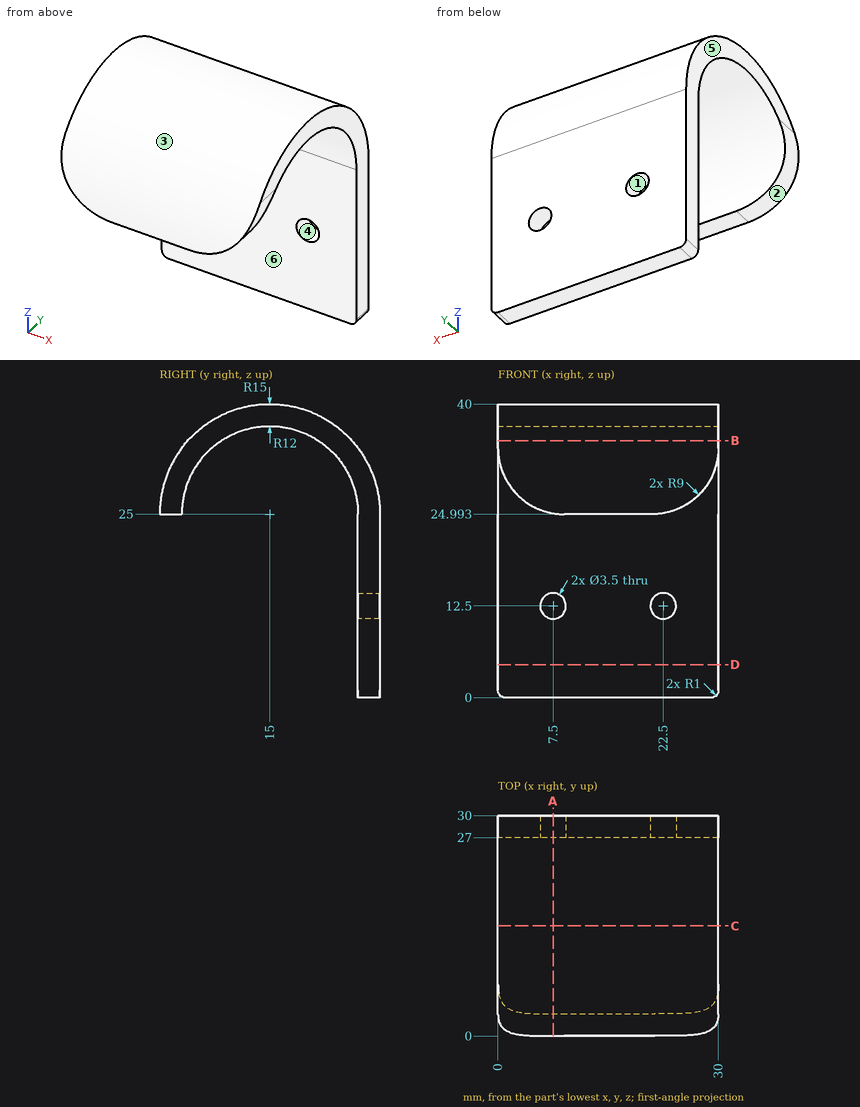
Source: three-view drawing plus pictorial views. Frame: mm from the lowest corner of the part. A direction names the side the tool comes from. Round coordinates to 2 decimals unless told otherwise and drop trailing zeros. Loops run counter-clockwise (first coordinate to the right, second up) from the corner with the lowest first, then second, coordinate; pieces in that order, holes last.
Q1. Pull-direction query (X, two-part tool) for the marked faces 1, 2, 3 and 4; classes: released by +X, released by -X, zero draft, split by the parting line, or undercut.
Q2. Section B-B on z = 35. Return loops of the section in (x, y).
Q3. Pin query (flat end, axial travel): P1, Ø12, axis at x = 24, z = 11.5, coming from the -Y side; P2, Ø1.5, axis at x = 15.5, y = 2, coming from the -Z side; P3, Ø1, axis at y = 25.5, z = 22, coming from the -X side; P4, Ø8, axis at x = 11.5, z = 35.5, coming from the -Y side. Return the tip coordinate at first contact, or that it passes through.
Q4. Section C-C on y = 15. Return loops of the section in (x, z).
Q5. Section A-A on x = 7.5. Return loops of the section in (y, z), plus the area to 3 significant figures.
Q6. Section D-D on z = 4.5. Return loops of the section in (x, y), plus the area to 3 significant figures.
Q7. Access query for the marked faces 5 and 6. Directions: +Z, -Z, +X, -X, +Y, -Y. A direction counts if a zero-diameter tool reaches every point of the face in a straight line with its end or side. Return the directions, or none.
Q8. Material intervals for L1, parallel to X at y = 28, z = 12.5; L2, parallel to Y at x = 24, z = 2.5; L3, parallel to Y at x = 12.5, z = 27, sorted ascending.
Evaluation:
1. face 1: undercut
1. face 2: released by -X
1. face 3: zero draft
1. face 4: undercut
2. outline: (0, 3.82) - (30, 3.82) - (30, 8.37) - (0, 8.37) - close; (0, 21.63) - (30, 21.63) - (30, 26.18) - (0, 26.18) - close
3. P1: stops at y = 27
3. P2: stops at z = 24.99
3. P3: passes through
3. P4: stops at y = 1.48
4. outline: (0, 37) - (30, 37) - (30, 40) - (0, 40) - close
5. outline: (0, 25.12) - (3, 25.12) arc R12 cw to (27, 25) - (27, 14.25) - (30, 14.25) - (30, 25) arc R15 ccw to start; (27, 0) - (30, 0) - (30, 10.75) - (27, 10.75) - close
5. area: 191 mm2
6. outline: (0, 27) - (30, 27) - (30, 30) - (0, 30) - close
6. area: 90.0 mm2
7. face 5: +Z, -Z, -X, +Y, -Y
7. face 6: -Z, +X, -X, -Y
8. L1: x = 0 to 5.75, 9.25 to 20.75, 24.25 to 30
8. L2: y = 27 to 30
8. L3: y = 0.13 to 3.17, 26.83 to 29.87
